Check sheet for the modelled part. Datum: model origin and axes. Units: mm. Give positions to 0.01 mm unless a question says otherwise; leave off trailing zeros. Write each loop counter-clockwise with the first axis right and the second up, starting at its lowest first coordinate (ties: lowest second). Pieces come first, ordered by that corner, then holes. Notation, with made-up numbers: M 63.25,52.5 L 81.25,52.5 A14 cw 81.25,65.5 Z; hole C -1,35 d2. An arc over 180 degrees is marked long. Use CSV: the item, a comma, the result in double quotes. Start each with the question number.
1. Mould release check, pull along Z, two halves, no side actions. Record for faces 1 (the face through (89.455, 2.348, 40.816)), 2 (the face through (31, 4.762, -52)): +Z half, -Z half, draft (parallel to the pull), parting line (faces both ways), or undercut.
2. Scan lines: line 1 (X direction, y = 3, z = 18); line 2 (X direction, y = 0.2, z = -27); line 3 (X direction, y = 2.85, z = -43.4). Record each from-to range of solid material in increasing order.
3. Cross-section at B-B, the plane x = -66.15. Enter the section's corners in (y, z).
4. Depth check by flat-ended pin: P1, Ø5.5, axis at x = 83.05, z = -73.3, coming from the -Y side. Enter the tip coordinate at first touch or a pass-through.
5. Cross-section at A-A, the plane x = 0. Enter the section's corners in (y, z), and give its area (3 significant figures).
6. Cross-section at C-C, the plane z = -43.4. Enter the section's corners in (x, y).
from build123d import *

# Parameters (mm, degrees)
SKETCH1_W           = 216.8
SKETCH1_H           = 260
SKETCH1_R           = 3.15
SKETCH1_R_2         = 2.5
SKETCH1_R_3         = 4.5
SKETCH1_R_4         = 2.8
SKETCH1_R_5         = 1.65
BOSS_EXTRUDE1_DEPTH = 4.7625


with BuildPart() as part:
    # Sketch1 → Boss-Extrude1 (new body)
    with BuildSketch(Plane(origin=(0, 0, 0), x_dir=(1, 0, 0), z_dir=(0, 1, 0))):
        with Locations((32.25, 49.916)):
            Rectangle(SKETCH1_W, SKETCH1_H)
        with Locations(Location((0, 0, 0), (0, 0, 90))):
            Circle(SKETCH1_R, mode=Mode.SUBTRACT)
        with Locations(Location((64.5, 27, 0), (0, 0, 90))):
            Circle(SKETCH1_R, mode=Mode.SUBTRACT)
        with Locations(Location((0, 43.4, 0), (0, 0, 90))):
            Circle(SKETCH1_R, mode=Mode.SUBTRACT)
        with Locations(Location((64.5, 70.4, 0), (0, 0, 90))):
            Circle(SKETCH1_R, mode=Mode.SUBTRACT)
        with Locations(Location((14.724, 125.484, 0), (0, 0, 90))):
            Circle(SKETCH1_R_2, mode=Mode.SUBTRACT)
        with Locations(Location((49.776, 125.484, 0), (0, 0, 90))):
            Circle(SKETCH1_R_2, mode=Mode.SUBTRACT)
        with Locations(Location((14.724, 88.4, 0), (0, 0, 90))):
            Circle(SKETCH1_R_2, mode=Mode.SUBTRACT)
        with Locations(Location((49.776, 88.4, 0), (0, 0, 90))):
            Circle(SKETCH1_R_2, mode=Mode.SUBTRACT)
        with Locations(Location((-20.963, 113.292, 0), (0, 0, 90))):
            Circle(SKETCH1_R_3, mode=Mode.SUBTRACT)
        with Locations(Location((85.463, 113.292, 0), (0, 0, 90))):
            Circle(SKETCH1_R_3, mode=Mode.SUBTRACT)
        with Locations(Location((14.724, -18, 0), (0, 0, 90))):
            Circle(SKETCH1_R_2, mode=Mode.SUBTRACT)
        with Locations(Location((49.776, -18, 0), (0, 0, 90))):
            Circle(SKETCH1_R_2, mode=Mode.SUBTRACT)
        with Locations(Location((14.724, -55.084, 0), (0, 0, 90))):
            Circle(SKETCH1_R_2, mode=Mode.SUBTRACT)
        with Locations(Location((49.776, -55.084, 0), (0, 0, 90))):
            Circle(SKETCH1_R_2, mode=Mode.SUBTRACT)
        with Locations(Location((-20.963, -42.892, 0), (0, 0, 90))):
            Circle(SKETCH1_R_3, mode=Mode.SUBTRACT)
        with Locations(Location((85.463, -42.892, 0), (0, 0, 90))):
            Circle(SKETCH1_R_3, mode=Mode.SUBTRACT)
        with Locations(Location((-66.15, 159.916, 0), (0, 0, 90))):
            Circle(SKETCH1_R_4, mode=Mode.SUBTRACT)
        with Locations(Location((-66.15, 49.916, 0), (0, 0, 90))):
            Circle(SKETCH1_R_4, mode=Mode.SUBTRACT)
        with Locations(Location((-66.15, -60.084, 0), (0, 0, 90))):
            Circle(SKETCH1_R_4, mode=Mode.SUBTRACT)
        with Locations(Location((130.65, -60.084, 0), (0, 0, 90))):
            Circle(SKETCH1_R_4, mode=Mode.SUBTRACT)
        with Locations(Location((130.65, 49.916, 0), (0, 0, 90))):
            Circle(SKETCH1_R_4, mode=Mode.SUBTRACT)
        with Locations(Location((130.65, 159.916, 0), (0, 0, 90))):
            Circle(SKETCH1_R_4, mode=Mode.SUBTRACT)
        with Locations(Location((-18.55, 73.3, 0), (0, 0, 90))):
            Circle(SKETCH1_R_5, mode=Mode.SUBTRACT)
        with Locations(Location((83.05, 73.3, 0), (0, 0, 90))):
            Circle(SKETCH1_R_5, mode=Mode.SUBTRACT)
        with Locations(Location((-18.55, -2.9, 0), (0, 0, 90))):
            Circle(SKETCH1_R_5, mode=Mode.SUBTRACT)
        with Locations(Location((83.05, -2.9, 0), (0, 0, 90))):
            Circle(SKETCH1_R_5, mode=Mode.SUBTRACT)
    extrude(amount=BOSS_EXTRUDE1_DEPTH)


solid = part.part
Worked answers:
1,face 1,"undercut"
1,face 2,"draft"
2,line 1,"x = -76.15 to 12.22, 17.22 to 47.28, 52.28 to 140.65"
2,line 2,"x = -76.15 to 61.35, 67.65 to 140.65"
2,line 3,"x = -76.15 to -3.15, 3.15 to 140.65"
3,outline,"M 0,-179.92 L 4.76,-179.92 L 4.76,-162.72 L 0,-162.72 Z; M 0,-157.12 L 4.76,-157.12 L 4.76,-52.72 L 0,-52.72 Z; M 0,-47.12 L 4.76,-47.12 L 4.76,57.28 L 0,57.28 Z; M 0,62.88 L 4.76,62.88 L 4.76,80.08 L 0,80.08 Z"
4,P1,"stops at y = 0"
5,outline,"M 0,-179.92 L 4.76,-179.92 L 4.76,-46.55 L 0,-46.55 Z; M 0,-40.25 L 4.76,-40.25 L 4.76,-3.15 L 0,-3.15 Z; M 0,3.15 L 4.76,3.15 L 4.76,80.08 L 0,80.08 Z"
5,area,"1,180 mm^2"
6,outline,"M -76.15,0 L -3.15,0 L -3.15,4.76 L -76.15,4.76 Z; M 3.15,0 L 140.65,0 L 140.65,4.76 L 3.15,4.76 Z"
